The listing builds one solid part. Answer for the finished solid, in the listing's coordinates (mm). A direction names the side the tool comes from. Coordinates: 2 decimals unless noted, no trailing zeros. Write each loop counter-clockwise with the first axis right and the second up, starting at its lowest first coordinate (ties: lowest second). Pieces come first, ordered by that corner, then holes.
from build123d import *

# Parameters (mm, degrees)
BOSS_EXTRUDE1_DEPTH     = 14.5
CUT_EXTRUDE2_DEPTH      = 36.864327681
CUT_EXTRUDE2_DEPTH_BACK = 36.864327681
SKETCH4_R               = 0.9
SKETCH4_W               = 11
SKETCH4_H               = 11
SKETCH5_R               = 1.25
SKETCH5_R_2             = 1.6
CUT_EXTRUDE3_DEPTH      = 34.797189232
FILLET1_R               = 3
CUT_EXTRUDE5_DEPTH      = 36.864327681
CUT_EXTRUDE5_DEPTH_BACK = 36.864327681


with BuildPart() as part:
    # Sketch1 → Boss-Extrude1 (new, symmetric)
    with BuildSketch(Plane(origin=(0, 0, 0), x_dir=(1, 0, 0), z_dir=(0, 1, 0))):
        Polygon((-7.131727984, 0), (-26, 0), (-26, -4), (-16, -4), (0, -20), (26, -20), (26, 0), (7.131727984, 0), (0, -7.131727984), align=None)
    extrude(amount=BOSS_EXTRUDE1_DEPTH, both=True)

    # Sketch4 → Cut-Extrude2 (cut, two sides: drawn at the far end of the back side and taken through both)
    with BuildSketch(Plane.XY.offset(20).offset(-CUT_EXTRUDE2_DEPTH_BACK)):
        with Locations((21, 10)):
            Circle(SKETCH4_R)
        with Locations((21, -10)):
            Circle(SKETCH4_R)
        with Locations((20.5, 0)):
            Rectangle(SKETCH4_W, SKETCH4_H)
    extrude(amount=CUT_EXTRUDE2_DEPTH + CUT_EXTRUDE2_DEPTH_BACK, mode=Mode.SUBTRACT)

    # Sketch5 → Cut-Extrude3 (cut, through all)
    with BuildSketch(Plane.XY.offset(4)):
        with Locations((-21, 10)):
            Circle(SKETCH5_R)
        with Locations((-21, -10)):
            Circle(SKETCH5_R_2)
    extrude(amount=-CUT_EXTRUDE3_DEPTH, mode=Mode.SUBTRACT)

    # Fillet1
    fillet1_edges = [part.edges().sort_by_distance(p)[0] for p in [
        (-16, 0, 4),
    ]]
    fillet(fillet1_edges, radius=FILLET1_R)

    # Sketch8 → Cut-Extrude5 (cut, two sides: drawn at the far end of the back side and taken through both)
    with BuildSketch(Plane(origin=(0, 0, 0), x_dir=(1, 0, 0), z_dir=(0, 1, 0)).offset(-CUT_EXTRUDE5_DEPTH_BACK)):
        Polygon((9.253048327, 0), (-9.253048327, 0), (0, -9.253048327), align=None)
    extrude(amount=CUT_EXTRUDE5_DEPTH + CUT_EXTRUDE5_DEPTH_BACK, mode=Mode.SUBTRACT)


solid = part.part
Q1. The part is cut by section C-C, the plane y = -10. Write down the section's boundary in (x, z).
Answers below:
outline: (-26, 0) - (-22.6, 0) - (-22.6, 4) - (-26, 4) - close; (-19.4, 0) - (-9.25, 0) - (0, 9.25) - (9.25, 0) - (20.1, 0) - (20.1, 20) - (0, 20) - (-15.12, 4.88) arc R3 cw to (-17.24, 4) - (-19.4, 4) - close; (21.9, 0) - (26, 0) - (26, 20) - (21.9, 20) - close
Q2. The part is cut by section B-B, the plane z = 2.75. Write down the section's boundary in (x, y), then the cut area to 3 significant figures.
Answers below:
outline: (-26, -14.5) - (-6.5, -14.5) - (-6.5, 14.5) - (-26, 14.5) - close; (6.5, -14.5) - (26, -14.5) - (26, -5.5) - (15, -5.5) - (15, 5.5) - (26, 5.5) - (26, 14.5) - (6.5, 14.5) - close; hole circle Ø3.2 at (-21, -10); hole circle Ø2.5 at (-21, 10); hole circle Ø1.8 at (21, -10); hole circle Ø1.8 at (21, 10)
area: 992 mm2
Q3. Find the intervals of material crossed by probe 1 along Y at (x, z) = (21, 9); probe 2 along Y at (x, z) = (-21, 1.3); probe 3 along Y at (x, z) = (20, 7.5), in increasing order.
Answers below:
probe 1: y = -14.5 to -10.9, -9.1 to -5.5, 5.5 to 9.1, 10.9 to 14.5
probe 2: y = -14.5 to -11.6, -8.4 to 8.75, 11.25 to 14.5
probe 3: y = -14.5 to -5.5, 5.5 to 14.5
Q4. Given pin 1 (12 mm diameter, centred on y = -2.5, z = 7.5, fed in from +X); pin 2 (4.5 mm diameter, centred on x = -23, y = -6.5, fed in from +Z); pin 3 (1 mm diameter, centred on y = 6.5, z = 14, fed in from -X); pin 4 (2.5 mm diameter, centred on x = -21, y = -10, fed in from -Z), each flat-ended and moving along its own axis, determine where each tip first touches the part or whether it passes through.
Answers below:
pin 1: stops at x = 26
pin 2: stops at z = 4
pin 3: stops at x = -6.5
pin 4: passes through
Q5. The part is cut by section A-A, the plane x = 21. Write down the section's boundary in (y, z), then the cut area to 3 significant figures.
Answers below:
outline: (-14.5, 0) - (-10.9, 0) - (-10.9, 20) - (-14.5, 20) - close; (-9.1, 0) - (-5.5, 0) - (-5.5, 20) - (-9.1, 20) - close; (5.5, 0) - (9.1, 0) - (9.1, 20) - (5.5, 20) - close; (10.9, 0) - (14.5, 0) - (14.5, 20) - (10.9, 20) - close
area: 288 mm2
Q6. Which of the six approach directions +Z, -Z, +X, -X, +Y, -Y give full straight-line access (tool end or side, diameter ignored) to faces 4 (the face through (5, -14.5, 10)), 5 (the face through (20, 5.5, 10)), 6 (the face through (-4.691, -0.203, 4.562)), 7 (the face through (-22, 0, 4))?
Answers below:
face 4: +Z, -Z, +X, -X, -Y
face 5: +Z, -Z, +X
face 6: -Z, +Y, -Y
face 7: +Z, -X, +Y, -Y
Q7. Determine the mould class of faces 1 (the face through (5, 14.5, 10)), 2 (the face through (26, -10, 10)), 3 (the face through (-20.328, 11.054, 2.028)) for opening direction Y: released by +Y, released by -Y, zero draft, split by the parting line, or undercut.
Answers below:
face 1: released by +Y
face 2: zero draft
face 3: undercut
Q8. The part is cut by section D-D, the plane x = -21. Write down the section's boundary in (y, z), then the cut area to 3 significant figures.
Answers below:
outline: (-14.5, 0) - (-11.6, 0) - (-11.6, 4) - (-14.5, 4) - close; (-8.4, 0) - (8.75, 0) - (8.75, 4) - (-8.4, 4) - close; (11.25, 0) - (14.5, 0) - (14.5, 4) - (11.25, 4) - close
area: 93.2 mm2
